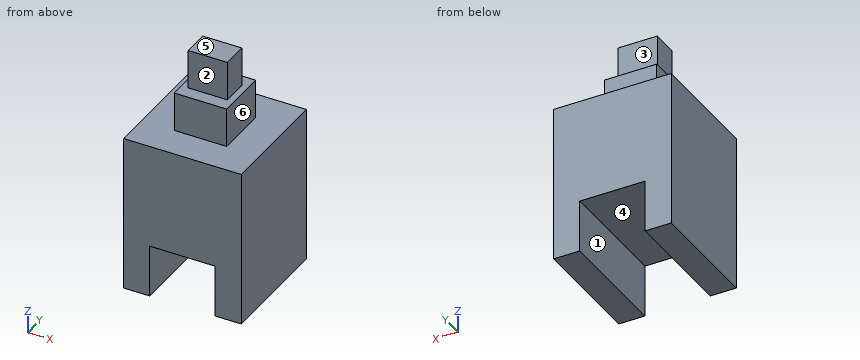
```python
from build123d import *

# Parameters (mm, degrees)
SKETCH1_W           = 9
SKETCH1_H           = 9
MAIN_BODY_DEPTH     = 8
SKETCH2_W           = 4
SKETCH2_H           = 4
BOSS_EXTRUDE2_DEPTH = 3
SKETCH3_W           = 3
SKETCH3_H           = 2
BOSS_EXTRUDE3_DEPTH = 3
SKETCH4_W           = 2
SKETCH4_H           = 9
PINS_DEPTH          = 4


with BuildPart() as part:
    # Sketch1 → MAIN BODY (new body)
    with BuildSketch(Plane.XY):
        Rectangle(SKETCH1_W, SKETCH1_H)
    extrude(amount=MAIN_BODY_DEPTH)

    # Sketch2 → Boss-Extrude2 (add)
    with BuildSketch(Plane.XY.offset(8)):
        Rectangle(SKETCH2_W, SKETCH2_H)
    extrude(amount=BOSS_EXTRUDE2_DEPTH)

    # Sketch3 → Boss-Extrude3 (add)
    with BuildSketch(Plane.XY.offset(11)):
        Rectangle(SKETCH3_W, SKETCH3_H)
    extrude(amount=BOSS_EXTRUDE3_DEPTH)

    # Sketch4 → PINS (add)
    with BuildSketch(Plane(origin=(0, 0, 0), x_dir=(-1, 0, 0), z_dir=(0, 0, -1))):
        with Locations((-3.5, 0)):
            Rectangle(SKETCH4_W, SKETCH4_H)
        with Locations((3.5, 0)):
            Rectangle(SKETCH4_W, SKETCH4_H)
    extrude(amount=PINS_DEPTH)


solid = part.part
```
Here's how the part is built. I have some questions about the finished solid (model axes, mm). Face numbers are marked on the shaded views. A direction names the side the tool comes from. Give positions to 0.01 mm unless a question says otherwise; leave off trailing zeros. Write each loop counter-clockwise with the first axis right and the second up, starting at its lowest first coordinate (ties: lowest second). Pieces come first, ordered by that corner, then holes. Notation, with made-up numbers: M 87.5,4.25 L 104.5,4.25 A21 ccw 104.5,10.25 Z; hole C 40,60 d4. An arc over 180 degrees is marked long. Put each result on its own line as item: value. Start each with the question number.
Item 1: Thinking about a two-plate mould opening in X: for the marked faces 4, 5 and 6, which applies, +X half, -X half, draft (parallel to the pull), parting line (faces both ways), or undercut?
Item 2: If we section it at C-C, the plane x = 0.25: Write out the boundary of the cut face in (y, z).
Item 3: If we section it at A-A, the plane z = -1.25: Write out the boundary of the cut face in (x, y), then the cut area to 3 significant figures.
Item 4: On a 3-axis mill with a long thin cutter (end or side, diameter ignored), from which of +Z, -Z, +X, -X, +Y, -Y can I reach the whole of each face in a straight line? I mean the marked faces 1, 2 and 3. Say none if no direction works.
Item 5: I need wall thicknesses on L1, parallel to Z at x = 0.75, y = -1.5; L2, parallel to Z at x = -3.5, y = 2.75; L3, parallel to Y at x = 0.25, z = 10.5. Which ranges of each line are inside material? Lowest first, please. Write a range as from..to.
Item 6: If we section it at B-B, the plane y = 3: Write out the boundary of the cut face in (x, z).
Item 7: If we section it at D-D, the plane y = -0.5: Write out the boundary of the cut face in (x, z).
Item 8: Will these pins go through, and if not, where does the flat tip stop? pin 1 (1 mm diameter, centred on y = 3, z = 12, fed in from +X); pin 2 (0.9 mm diameter, centred on x = -0.5, z = 10, fed in from +Y); pin 3 (2 mm diameter, centred on y = 0, z = 12.5, fed in from +X); pin 4 (2.5 mm diameter, centred on y = 0.5, z = 10, fed in from +X).
Values:
1. face 4: undercut
1. face 5: draft
1. face 6: +X half
2. outline: M -4.5,0 L 4.5,0 L 4.5,8 L 2,8 L 2,11 L 1,11 L 1,14 L -1,14 L -1,11 L -2,11 L -2,8 L -4.5,8 Z
3. outline: M -4.5,-4.5 L -2.5,-4.5 L -2.5,4.5 L -4.5,4.5 Z; M 2.5,-4.5 L 4.5,-4.5 L 4.5,4.5 L 2.5,4.5 Z
3. area: 36.0 mm²
4. face 1: -Z, +Y, -Y
4. face 2: +Z, +X, -X, -Y
4. face 3: +Z, +X, -X, +Y
5. L1: 0..11
5. L2: -4..8
5. L3: -2..2
6. outline: M -4.5,-4 L -2.5,-4 L -2.5,0 L 2.5,0 L 2.5,-4 L 4.5,-4 L 4.5,8 L -4.5,8 Z
7. outline: M -4.5,-4 L -2.5,-4 L -2.5,0 L 2.5,0 L 2.5,-4 L 4.5,-4 L 4.5,8 L 2,8 L 2,11 L 1.5,11 L 1.5,14 L -1.5,14 L -1.5,11 L -2,11 L -2,8 L -4.5,8 Z
8. pin 1: through
8. pin 2: y = 2
8. pin 3: x = 1.5
8. pin 4: x = 2
